Verification items for the finished model (mm, model axes). A direction names the side the tool comes from. Give positions to 0.01 mm unless a question says otherwise; leave off trailing zeros. Write each loop counter-clockwise with the first axis right and the second up, starting at its lowest first coordinate (ties: lowest second). Pieces come first, ordered by that corner, then holes. Notation, with made-up numbers: (-20.75, -27) -> (8.25, -27) arc R20 ccw to (8.25, -2) -> close; hole circle Ø11 at (9.5, 62). An arc over 180 degrees is marked (long way). Answer as CSV lines item,"result".
```python
from build123d import *

# Parameters (mm, degrees)
SKETCH1_W               = 40
SKETCH1_H               = 40
BOSS_EXTRUDE1_DEPTH     = 4
SKETCH2_R               = 2
CUT_EXTRUDE1_DEPTH      = 29.565713714
CUT_EXTRUDE2_DEPTH      = 29.565713714
SKETCH4_W               = 15.5
SKETCH4_H               = 4
SKETCH4_W_2             = 4
SKETCH4_H_2             = 15.5
BOSS_EXTRUDE2_DEPTH     = 8
CUT_EXTRUDE3_DEPTH      = 43.895221179
CUT_EXTRUDE3_DEPTH_BACK = 5
SKETCH5_R               = 2
CUT_EXTRUDE4_DEPTH      = 43.895221179
CUT_EXTRUDE4_DEPTH_BACK = 5
SKETCH6_R               = 2
SKETCH7_R               = 3
CUT_EXTRUDE5_DEPTH      = 2
CIRPATTERN1_COUNT       = 4
CHAMFER1_SIZE           = 1
FILLET1_R               = 1
CHAMFER2_SIZE           = 1
SKETCH10_R              = 3.5
CUT_EXTRUDE6_DEPTH      = 2


with BuildPart() as part:
    # Sketch1 → Boss-Extrude1 (new body)
    with BuildSketch(Plane(origin=(0, 0, 0), x_dir=(1, 0, 0), z_dir=(0, 1, 0))):
        Rectangle(SKETCH1_W, SKETCH1_H)
    extrude(amount=BOSS_EXTRUDE1_DEPTH)

    # Sketch2 → Cut-Extrude1 (cut, through all)
    with BuildSketch(Plane(origin=(0, 4, 0), x_dir=(1, 0, 0), z_dir=(0, 1, 0))):
        with Locations(Location((-10, 0, 0), (0, 0, 270))):
            Circle(SKETCH2_R)
        with Locations(Location((0, 10, 0), (0, 0, 270))):
            Circle(SKETCH2_R)
        with Locations(Location((10, 0, 0), (0, 0, 270))):
            Circle(SKETCH2_R)
        with Locations(Location((0, -10, 0), (0, 0, 270))):
            Circle(SKETCH2_R)
    extrude(amount=-CUT_EXTRUDE1_DEPTH, mode=Mode.SUBTRACT)

    # Sketch3 → Cut-Extrude2 (cut, through all)
    with BuildSketch(Plane(origin=(0, 4, 0), x_dir=(1, 0, 0), z_dir=(0, 1, 0))):
        Polygon((-7.75, 20), (-20, 20), (-20, 7.75), align=None)
        Polygon((20, 7.75), (20, 20), (7.75, 20), align=None)
        Polygon((20, -7.75), (7.75, -20), (20, -20), align=None)
        Polygon((-20, -7.75), (-7.75, -20), (-20, -20), align=None)
    extrude(amount=-CUT_EXTRUDE2_DEPTH, mode=Mode.SUBTRACT)

    # Sketch4 → Boss-Extrude2 (add)
    with BuildSketch(Plane(origin=(0, 4, 0), x_dir=(1, 0, 0), z_dir=(0, 1, 0))):
        with Locations((0, 18)):
            Rectangle(SKETCH4_W, SKETCH4_H)
        with Locations((18, 0)):
            Rectangle(SKETCH4_W_2, SKETCH4_H_2)
        with Locations((0, -18)):
            Rectangle(SKETCH4_W, SKETCH4_H)
        with Locations((-18, 0)):
            Rectangle(SKETCH4_W_2, SKETCH4_H_2)
    extrude(amount=BOSS_EXTRUDE2_DEPTH)

    # Sketch5 → Cut-Extrude3 (cut, two sides: drawn at the far end of the back side and taken through both)
    with BuildSketch(Plane.ZY.offset(-16).offset(-CUT_EXTRUDE3_DEPTH_BACK)):
        with Locations((0, 8)):
            Circle(SKETCH5_R)
    extrude(amount=CUT_EXTRUDE3_DEPTH + CUT_EXTRUDE3_DEPTH_BACK, mode=Mode.SUBTRACT)

    # Sketch6 → Cut-Extrude4 (cut, two sides: drawn at the far end of the back side and taken through both)
    with BuildSketch(Plane(origin=(0, 0, 16), x_dir=(-1, 0, 0), z_dir=(0, 0, -1)).offset(-CUT_EXTRUDE4_DEPTH_BACK)):
        with Locations(Location((0, 8, 0), (0, 0, 180))):
            Circle(SKETCH6_R)
    extrude(amount=CUT_EXTRUDE4_DEPTH + CUT_EXTRUDE4_DEPTH_BACK, mode=Mode.SUBTRACT)

    # Sketch7 → Cut-Extrude5 (cut)
    with BuildSketch(Plane.XY.offset(20)):
        with Locations((0, 8)):
            Circle(SKETCH7_R)
    cut_extrude5 = extrude(amount=-CUT_EXTRUDE5_DEPTH, mode=Mode.SUBTRACT)

    # CirPattern1: Cut-Extrude5 ×4 about axis
    cirpattern1_axis = Axis((0, 0, 0), (0, 1, 0))
    for i in range(1, CIRPATTERN1_COUNT):
        add(cut_extrude5.rotate(cirpattern1_axis, i * 360 / CIRPATTERN1_COUNT), mode=Mode.SUBTRACT)

    # Chamfer1
    chamfer1_edges = [part.edges().sort_by_distance(p)[0] for p in [
        (7.75, 12, 18),
        (-7.75, 12, 18),
        (-18, 12, 7.75),
        (-18, 12, -7.75),
        (20, 0, 0),
        (0, 0, 20),
        (-20, 0, 0),
        (0, 0, -20),
        (-13.875, 0, 13.875),
        (13.875, 0, 13.875),
        (13.875, 0, -13.875),
        (-13.875, 0, -13.875),
        (7.75, 12, -18),
        (-7.75, 12, -18),
        (18, 12, -7.75),
        (18, 12, 7.75),
    ]]
    chamfer(chamfer1_edges, length=CHAMFER1_SIZE)

    # Fillet1
    fillet1_edges = [part.edges().sort_by_distance(p)[0] for p in [
        (-3, 8, 18),
        (-18, 8, -3),
        (3, 8, -18),
        (18, 8, 3),
    ]]
    fillet(fillet1_edges, radius=FILLET1_R - 0.0001)  # a hair under: the kernel refuses the full size

    # Chamfer2
    chamfer2_edges = [part.edges().sort_by_distance(p)[0] for p in [
        (0, 4, 16),
        (-16, 4, 0),
        (-13.875, 4, 13.875),
        (13.875, 4, 13.875),
        (13.875, 4, -13.875),
        (-13.875, 4, -13.875),
        (0, 4, -16),
        (16, 4, 0),
    ]]
    chamfer(chamfer2_edges, length=CHAMFER2_SIZE)

    # Sketch10 → Cut-Extrude6 (cut)
    with BuildSketch(Plane(origin=(0, 4, 0), x_dir=(1, 0, 0), z_dir=(0, 1, 0))):
        with Locations(Location((-10, 0, 0), (0, 0, 270))):
            Circle(SKETCH10_R)
        with Locations(Location((0, 10, 0), (0, 0, 270))):
            Circle(SKETCH10_R)
        with Locations(Location((10, 0, 0), (0, 0, 270))):
            Circle(SKETCH10_R)
        with Locations(Location((0, -10, 0), (0, 0, 270))):
            Circle(SKETCH10_R)
    extrude(amount=-CUT_EXTRUDE6_DEPTH, mode=Mode.SUBTRACT)


solid = part.part
```
1) Scan lines: line 1 along Y through (x, z) = (0, -16.75); line 2 along Z through (x, y) = (-16.95, 8); line 3 along X through (y, z) = (5.25, 7). Record each from-to range of solid material in increasing order.
Reported:
line 1,"0 to 6, 10 to 12"
line 2,"-7.75 to -2, 2 to 7.75"
line 3,"-20 to -16, 16 to 20"
2) Draft check along Z on faces 1 (the cylindrical face through (0.154, 3.014, 6.503)), 2 (the flat face through (13.96, 2.01, 13.79)), 3 (the flat face through (18, 7, -7.75)). Enter one of: +Z half, -Z half, draft (parallel to the pull), parting line (faces both ways), or undercut.
Reported:
face 1,"undercut"
face 2,"+Z half"
face 3,"-Z half"
3) Section check C-C (z = -10). Record the boundary of the cut face in (x, y), and give its area (3 significant figures).
Reported:
outline,"(-17.75, 1) -> (-16.34, 0) -> (-2, 0) -> (-2, 2) -> (-3.5, 2) -> (-3.5, 4) -> (-16.34, 4) -> (-17.75, 3) -> close; (2, 0) -> (16.34, 0) -> (17.75, 1) -> (17.75, 3) -> (16.34, 4) -> (3.5, 4) -> (3.5, 2) -> (2, 2) -> close"
area,"117 mm²"
4) Tool access check on faces 4 (the cylindrical face through (-1.2, 1, -11.6)), 5 (the flat face through (-12, 2, 2)). Record the directions out of +Z, -Z, +X, -X, +Y, -Y that give a thin tool (end or side, any length) a straight path to the whole face; none if there is none.
Reported:
face 4,"+Y, -Y"
face 5,"+Y"
5) Section check A-A (x = -10). Record the boundary of the cut face in (y, z).
Reported:
outline,"(0, -16.34) -> (1, -17.75) -> (3, -17.75) -> (4, -16.34) -> (4, -3.5) -> (2, -3.5) -> (2, -2) -> (0, -2) -> close; (0, 2) -> (2, 2) -> (2, 3.5) -> (4, 3.5) -> (4, 16.34) -> (3, 17.75) -> (1, 17.75) -> (0, 16.34) -> close"
6) Section check D-D (x = 5). Record the boundary of the cut face in (y, z).
Reported:
outline,"(0, -19) -> (1, -20) -> (12, -20) -> (12, -16) -> (5, -16) -> (4, -15) -> (4, 15) -> (5, 16) -> (12, 16) -> (12, 20) -> (1, 20) -> (0, 19) -> close"
7) Depth check by flat-ended pin: pin 1 (10 mm diameter, centred on x = -4.5, z = 10.5, fed in from +Y); pin 2 (5 mm diameter, centred on x = 0, y = 8, fed in from -Z); pin 3 (1 mm diameter, centred on x = -2, z = -10.5, fed in from +Y); pin 4 (2 mm diameter, centred on x = -14, y = 8, fed in from +Z). Enter the tip coordinate at first touch or a pass-through.
Reported:
pin 1,"y = 4.5"
pin 2,"z = -18.13"
pin 3,"y = 2"
pin 4,"through"
8) Section check B-B (z = 4.5). Record the boundary of the cut face in (x, y).
Reported:
outline,"(-20, 1) -> (-19, 0) -> (19, 0) -> (20, 1) -> (20, 12) -> (16, 12) -> (16, 5) -> (15, 4) -> (-15, 4) -> (-16, 5) -> (-16, 12) -> (-20, 12) -> close"
